Design review of the part built by this model. Coordinates are the model's own, in mm. Coordinates: 2 decimals unless noted, no trailing zeros. Loops run counter-clockwise (first coordinate to the right, second up) from the corner with the lowest first, then second, coordinate; pieces in that order, holes last.
Q1. For P1, Ø6.5, axis at x = 16, y = 20.5, coming from the -Z side, flat-tipped, find the tip position at first contact; note if it passes through.
Q2. Add section A-A on x = 87. Give the boundary of the cut face in (y, z), and give its area (3 significant figures).
Q3. Wall thickness on probe 1 along Y at (x, z) = (87, 1.7); probe 2 along Y at (x, z) = (85, 2.4): over which ranges is each line inside the solid? List them lowest first.
Q4. Add section B-B on z = 3.1. Give the boundary of the cut face in (x, y).
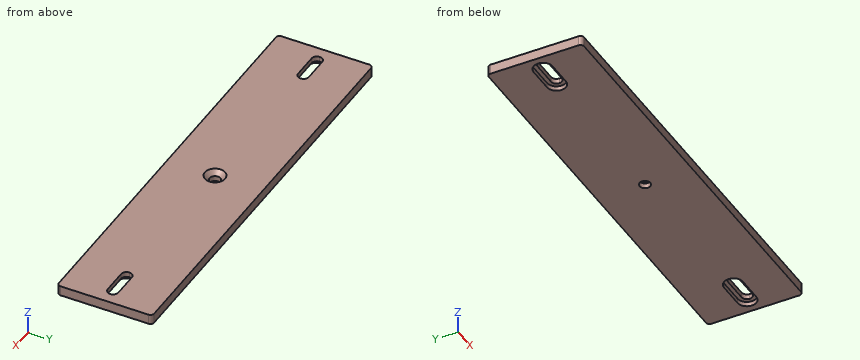
```python
from build123d import *

# Parameters (mm, degrees)
F0_W     = 174
F0_H     = 40
F0_R     = 2.25
F1_DEPTH = 4.2
F3_DEPTH = 2
F4_SIZE  = 2
F5_R     = 1.5


with BuildPart() as f1:
    # F0 (on Top) → F1 (new body)
    with BuildSketch(Plane.XY):
        with Locations((87, 20)):
            Rectangle(F0_W, F0_H)
        with BuildLine():
            ThreePointArc((4.5, 20), (5.15901, 21.59099), (6.75, 22.25))
            Line((6.75, 22.25), (17.25, 22.25))
            ThreePointArc((17.25, 22.25), (18.84099, 21.59099), (19.5, 20))
            ThreePointArc((19.5, 20), (18.84099, 18.40901), (17.25, 17.75))
            Line((17.25, 17.75), (6.75, 17.75))
            ThreePointArc((6.75, 17.75), (5.15901, 18.40901), (4.5, 20))
        make_face(mode=Mode.SUBTRACT)
        with Locations((87, 20)):
            Circle(F0_R, mode=Mode.SUBTRACT)
        with BuildLine():
            Line((156.75, 22.25), (167.25, 22.25))
            ThreePointArc((167.25, 22.25), (168.84099, 21.59099), (169.5, 20))
            ThreePointArc((169.5, 20), (168.84099, 18.40901), (167.25, 17.75))
            Line((167.25, 17.75), (156.75, 17.75))
            ThreePointArc((156.75, 17.75), (155.15901, 18.40901), (154.5, 20))
            ThreePointArc((154.5, 20), (155.15901, 21.59099), (156.75, 22.25))
        make_face(mode=Mode.SUBTRACT)
    extrude(amount=F1_DEPTH)

    # F2 (on Top) → F3 (cut)
    with BuildSketch(Plane.XY):
        with BuildLine():
            ThreePointArc((6.75, 23.95), (2.8, 20), (6.75, 16.05))
            Line((6.75, 16.05), (17.25, 16.05))
            ThreePointArc((17.25, 16.05), (21.2, 20), (17.25, 23.95))
            Line((17.25, 23.95), (6.75, 23.95))
        make_face()
        with BuildLine():
            Line((156.75, 16.05), (167.25, 16.05))
            ThreePointArc((167.25, 16.05), (171.2, 20), (167.25, 23.95))
            Line((167.25, 23.95), (156.75, 23.95))
            ThreePointArc((156.75, 23.95), (152.8, 20), (156.75, 16.05))
        make_face()
    extrude(amount=F3_DEPTH, mode=Mode.SUBTRACT)

    # F4
    f4_edges = [f1.edges().sort_by_distance(p)[0] for p in [
        (84.75, 20, 4.2),
    ]]
    chamfer(f4_edges, length=F4_SIZE)

    # F5
    f5_edges = [f1.edges().sort_by_distance(p)[0] for p in [
        (174, 0, 2.1),
        (174, 40, 2.1),
        (0, 40, 2.1),
        (0, 0, 2.1),
    ]]
    fillet(f5_edges, radius=F5_R)


solid = f1.part
```
Entries:
1. P1: stops at z = 2
2. outline: (0, 0) - (17.75, 0) - (17.75, 2.2) - (15.75, 4.2) - (0, 4.2) - close; (22.25, 0) - (40, 0) - (40, 4.2) - (24.25, 4.2) - (22.25, 2.2) - close
2. area: 145 mm2
3. probe 1: y = 0 to 17.75, 22.25 to 40
3. probe 2: y = 0 to 18.58, 21.42 to 40
4. outline: (0, 1.5) arc R1.5 ccw to (1.5, 0) - (172.5, 0) arc R1.5 ccw to (174, 1.5) - (174, 38.5) arc R1.5 ccw to (172.5, 40) - (1.5, 40) arc R1.5 ccw to (0, 38.5) - close; hole (4.5, 20) arc R2.25 ccw to (6.75, 17.75) - (17.25, 17.75) arc R2.25 ccw to (19.5, 20) arc R2.25 ccw to (17.25, 22.25) - (6.75, 22.25) arc R2.25 ccw to start; hole circle Ø6.3 at (87, 20); hole (154.5, 20) arc R2.25 ccw to (156.75, 17.75) - (167.25, 17.75) arc R2.25 ccw to (169.5, 20) arc R2.25 ccw to (167.25, 22.25) - (156.75, 22.25) arc R2.25 ccw to start
